Work out the finished part from the listing and answer in its coordinate system (mm). Round coordinates to 2 decimals unless told otherwise and drop trailing zeros. Write each loop counter-clockwise with the first axis right and the second up, starting at its lowest first coordinate (ties: lowest second). Pieces come first, ordered by that corner, then holes.
1. Find section C-C (y = 2.25). Write down the section's boundary in (x, z) (3 decimals), and give its area (3 significant figures).
2. Find section B-B (x = -2.5). Write down the section's boundary in (y, z) (3 decimals), and give its area (3 significant figures).
3. Straight lines are drawn through the part: probe 1 along X at (y, z) = (-1, 0.1); probe 2 along X at (y, z) = (5, 0.15) (3 decimals); probe 3 along Y at (x, z) = (0, -1.1). For each, find the intervals that lie inside material, in ascending order.
4. Find section D-D (z = -0.5). Write down the section's boundary in (x, y) (3 decimals).
5. Find section A-A (y = -0.5). Write down the section's boundary in (x, z) (3 decimals).
6. Flat-ended cylindrical pins translate along their axes: pin 1 Ø0.7 at (x, y) = (2.5, -2) entering from -Z (3 decimals); pin 2 Ø0.7 at (x, z) = (2.5, 0) entering from +Y (3 decimals). Find the tip coordinate at first contact, or state that the pin passes through.
```python
from build123d import *

# Parameters (mm, degrees)
SKETCH1_W           = 38.1
SKETCH1_H           = 2.4
BOSS_EXTRUDE1_DEPTH = 8.5
SKETCH2_W           = 0.63
SKETCH2_H           = 0.63
CUT_EXTRUDE1_DEPTH  = 6.5
SKETCH3_W           = 0.6
SKETCH3_H           = 0.35
BOSS_EXTRUDE2_DEPTH = 2.9
CHAMFER1_SIZE       = 0.4
SKETCH4_W           = 19.378829163
SKETCH4_H           = 4.471478983
CUT_EXTRUDE2_DEPTH  = 23.232914789
SKETCH7_W           = 15.24
SKETCH7_H           = 12.363721619
CUT_EXTRUDE3_DEPTH  = 21.997916563


with BuildPart() as part:
    # Sketch1 → Boss-Extrude1 (new body)
    with BuildSketch(Plane(origin=(0, 0, 0), x_dir=(1, 0, 0), z_dir=(0, 1, 0))):
        Rectangle(SKETCH1_W, SKETCH1_H)
    extrude(amount=BOSS_EXTRUDE1_DEPTH)

    # Sketch2 → Cut-Extrude1 (cut)
    with BuildSketch(Plane(origin=(0, 8.5, 0), x_dir=(1, 0, 0), z_dir=(0, 1, 0))):
        with Locations((-15.24, 0)):
            Rectangle(SKETCH2_W, SKETCH2_H)
        with Locations((-17.78, 0)):
            Rectangle(SKETCH2_W, SKETCH2_H)
        with Locations((-12.7, 0)):
            Rectangle(SKETCH2_W, SKETCH2_H)
        with Locations((-10.16, 0)):
            Rectangle(SKETCH2_W, SKETCH2_H)
        with Locations((-7.62, 0)):
            Rectangle(SKETCH2_W, SKETCH2_H)
        with Locations((-5.08, 0)):
            Rectangle(SKETCH2_W, SKETCH2_H)
        with Locations((-2.54, 0)):
            Rectangle(SKETCH2_W, SKETCH2_H)
        Rectangle(SKETCH2_W, SKETCH2_H)
        with Locations((2.54, 0)):
            Rectangle(SKETCH2_W, SKETCH2_H)
        with Locations((5.08, 0)):
            Rectangle(SKETCH2_W, SKETCH2_H)
        with Locations((7.62, 0)):
            Rectangle(SKETCH2_W, SKETCH2_H)
        with Locations((10.16, 0)):
            Rectangle(SKETCH2_W, SKETCH2_H)
        with Locations((12.7, 0)):
            Rectangle(SKETCH2_W, SKETCH2_H)
        with Locations((15.24, 0)):
            Rectangle(SKETCH2_W, SKETCH2_H)
        with Locations((17.78, 0)):
            Rectangle(SKETCH2_W, SKETCH2_H)
    extrude(amount=-CUT_EXTRUDE1_DEPTH, mode=Mode.SUBTRACT)

    # Sketch3 → Boss-Extrude2 (add)
    with BuildSketch(Plane.XZ):
        with Locations((-15.24, 0)):
            Rectangle(SKETCH3_W, SKETCH3_H)
        with Locations((-17.78, 0)):
            Rectangle(SKETCH3_W, SKETCH3_H)
        with Locations((-12.7, 0)):
            Rectangle(SKETCH3_W, SKETCH3_H)
        with Locations((-10.16, 0)):
            Rectangle(SKETCH3_W, SKETCH3_H)
        with Locations((-7.62, 0)):
            Rectangle(SKETCH3_W, SKETCH3_H)
        with Locations((-5.08, 0)):
            Rectangle(SKETCH3_W, SKETCH3_H)
        with Locations((-2.54, 0)):
            Rectangle(SKETCH3_W, SKETCH3_H)
        Rectangle(SKETCH3_W, SKETCH3_H)
        with Locations((2.54, 0)):
            Rectangle(SKETCH3_W, SKETCH3_H)
        with Locations((5.08, 0)):
            Rectangle(SKETCH3_W, SKETCH3_H)
        with Locations((7.62, 0)):
            Rectangle(SKETCH3_W, SKETCH3_H)
        with Locations((10.16, 0)):
            Rectangle(SKETCH3_W, SKETCH3_H)
        with Locations((12.7, 0)):
            Rectangle(SKETCH3_W, SKETCH3_H)
        with Locations((15.24, 0)):
            Rectangle(SKETCH3_W, SKETCH3_H)
        with Locations((17.78, 0)):
            Rectangle(SKETCH3_W, SKETCH3_H)
    extrude(amount=BOSS_EXTRUDE2_DEPTH)

    # Chamfer1
    chamfer1_edges = [part.edges().sort_by_distance(p)[0] for p in [
        (2.855, 8.5, 0),
        (2.54, 8.5, -0.315),
        (2.225, 8.5, 0),
        (2.54, 8.5, 0.315),
        (5.395, 8.5, 0),
        (5.08, 8.5, -0.315),
        (4.765, 8.5, 0),
        (5.08, 8.5, 0.315),
        (7.935, 8.5, 0),
        (7.62, 8.5, -0.315),
        (7.305, 8.5, 0),
        (7.62, 8.5, 0.315),
        (10.475, 8.5, 0),
        (10.16, 8.5, -0.315),
        (9.845, 8.5, 0),
        (10.16, 8.5, 0.315),
        (13.015, 8.5, 0),
        (12.7, 8.5, -0.315),
        (12.385, 8.5, 0),
        (12.7, 8.5, 0.315),
        (15.555, 8.5, 0),
        (15.24, 8.5, -0.315),
        (14.925, 8.5, 0),
        (15.24, 8.5, 0.315),
        (18.095, 8.5, 0),
        (17.78, 8.5, -0.315),
        (17.465, 8.5, 0),
        (17.78, 8.5, 0.315),
        (-17.465, 8.5, 0),
        (-17.78, 8.5, -0.315),
        (-18.095, 8.5, 0),
        (-17.78, 8.5, 0.315),
        (-14.925, 8.5, 0),
        (-15.24, 8.5, -0.315),
        (-15.555, 8.5, 0),
        (-15.24, 8.5, 0.315),
        (-12.385, 8.5, 0),
        (-12.7, 8.5, -0.315),
        (-13.015, 8.5, 0),
        (-12.7, 8.5, 0.315),
        (-9.845, 8.5, 0),
        (-10.16, 8.5, -0.315),
        (-10.475, 8.5, 0),
        (-10.16, 8.5, 0.315),
        (-7.305, 8.5, 0),
        (-7.62, 8.5, -0.315),
        (-7.935, 8.5, 0),
        (-7.62, 8.5, 0.315),
        (-4.765, 8.5, 0),
        (-5.08, 8.5, -0.315),
        (-5.395, 8.5, 0),
        (-5.08, 8.5, 0.315),
        (-2.225, 8.5, 0),
        (-2.54, 8.5, -0.315),
        (-2.855, 8.5, 0),
        (-2.54, 8.5, 0.315),
        (0.315, 8.5, 0),
        (0, 8.5, -0.315),
        (-0.315, 8.5, 0),
        (0, 8.5, 0.315),
    ]]
    chamfer(chamfer1_edges, length=CHAMFER1_SIZE)

    # Sketch4 → Cut-Extrude2 (cut, through all)
    with BuildSketch(Plane(origin=(0, 8.5, 0), x_dir=(1, 0, 0), z_dir=(0, 1, 0))):
        with Locations((16.039414582, -0.096925096)):
            Rectangle(SKETCH4_W, SKETCH4_H)
    extrude(amount=-CUT_EXTRUDE2_DEPTH, mode=Mode.SUBTRACT)

    # Sketch7 → Cut-Extrude3 (cut, through all)
    with BuildSketch(Plane.XY.offset(1.2)):
        with Locations((-11.43, 2.318139191)):
            Rectangle(SKETCH7_W, SKETCH7_H)
    extrude(amount=-CUT_EXTRUDE3_DEPTH, mode=Mode.SUBTRACT)


solid = part.part
```
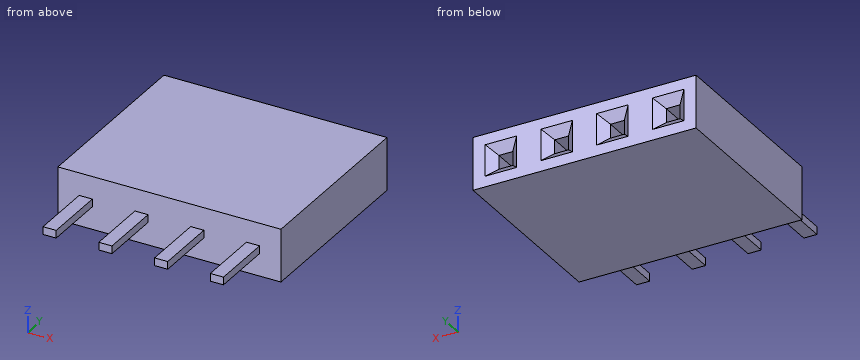
Worked answers:
1. outline: (-3.81, -1.2) - (6.35, -1.2) - (6.35, 1.2) - (-3.81, 1.2) - close; hole (-2.855, -0.315) - (-2.225, -0.315) - (-2.225, 0.315) - (-2.855, 0.315) - close; hole (-0.315, -0.315) - (0.315, -0.315) - (0.315, 0.315) - (-0.315, 0.315) - close; hole (2.225, -0.315) - (2.855, -0.315) - (2.855, 0.315) - (2.225, 0.315) - close; hole (4.765, -0.315) - (5.395, -0.315) - (5.395, 0.315) - (4.765, 0.315) - close
1. area: 22.8 mm2
2. outline: (-2.9, -0.175) - (0, -0.175) - (0, -1.2) - (8.5, -1.2) - (8.5, -0.715) - (8.1, -0.315) - (2, -0.315) - (2, 0.315) - (8.1, 0.315) - (8.5, 0.715) - (8.5, 1.2) - (0, 1.2) - (0, 0.175) - (-2.9, 0.175) - close
2. area: 17.2 mm2
3. probe 1: x = -2.84 to -2.24, -0.3 to 0.3, 2.24 to 2.84, 4.78 to 5.38
3. probe 2: x = -3.81 to -2.855, -2.225 to -0.315, 0.315 to 2.225, 2.855 to 4.765, 5.395 to 6.35
3. probe 3: y = 0 to 8.5
4. outline: (-3.81, 0) - (6.35, 0) - (6.35, 8.5) - (5.795, 8.5) - (5.58, 8.285) - (4.58, 8.285) - (4.365, 8.5) - (3.255, 8.5) - (3.04, 8.285) - (2.04, 8.285) - (1.825, 8.5) - (0.715, 8.5) - (0.5, 8.285) - (-0.5, 8.285) - (-0.715, 8.5) - (-1.825, 8.5) - (-2.04, 8.285) - (-3.04, 8.285) - (-3.255, 8.5) - (-3.81, 8.5) - close
5. outline: (-2.84, -0.175) - (-2.24, -0.175) - (-2.24, 0.175) - (-2.84, 0.175) - close; (-0.3, -0.175) - (0.3, -0.175) - (0.3, 0.175) - (-0.3, 0.175) - close; (2.24, -0.175) - (2.84, -0.175) - (2.84, 0.175) - (2.24, 0.175) - close; (4.78, -0.175) - (5.38, -0.175) - (5.38, 0.175) - (4.78, 0.175) - close
6. pin 1: stops at z = -0.175
6. pin 2: stops at y = 8.175
